The listing builds one solid part. Answer for the finished solid, in the listing's coordinates (mm). A direction names the side the tool comes from. Give positions to 0.01 mm unless a question says otherwise; leave off trailing zeros. Write each loop counter-clockwise with the first axis right and the second up, starting at its lowest first coordinate (ties: lowest second). Pieces come first, ordered by that corner, then holes. Notation, with made-up numbers: (4.5, 61.25) - (42.5, 61.25) arc R7 ccw to (42.5, 74.25) - close; hole circle Ø5 at (56, -21). An arc over 180 degrees is marked (long way). Answer in a Markdown table with one row per item. Add a question column.
from build123d import *

# Parameters (mm, degrees)
F1_DEPTH = 5
F3_DEPTH = 335
F4_W     = 5
F4_H     = 335
F5_DEPTH = 319
F7_DEPTH = 335


with BuildPart() as f1:
    # F0 (on Top) → F1 (new body)
    with BuildSketch(Plane.XY):
        Polygon((-324, 0), (0, 0), (0, 195), (-199, 195), (-199, 5), (-299, 5), (-319, 25), (-319, 195), (-324, 195), align=None)
    extrude(amount=F1_DEPTH)

    # F2 (on face) → F3 (join)
    with BuildSketch(Plane(origin=(0, 0, 0), x_dir=(1, 0, 0), z_dir=(0, 0, -1))):
        Polygon((-319, 0), (-324, 0), (-324, -195), (-319, -195), (-319, -25), align=None)
    extrude(amount=F3_DEPTH)

    # F4 (on face) → F5 (join, through all)
    with BuildSketch(Plane.YZ.offset(-319)):
        with Locations((2.5, -167.5)):
            Rectangle(F4_W, F4_H)
    extrude(amount=F5_DEPTH)

    # F6 (on face) → F7 (join, through all)
    with BuildSketch(Plane(origin=(0, 0, 0), x_dir=(1, 0, 0), z_dir=(0, 0, -1))):
        Polygon((0, -195), (0, -5), (-5, -5), (-5, -190), (-199, -190), (-199, -195), align=None)
    extrude(amount=F7_DEPTH)


solid = f1.part
1. Straight lines are drawn through the part: L1, parallel to X at y = 41.5, z = -220; L2, parallel to Y at x = -24, z = -287.5; L3, parallel to Z at x = -29, y = 83.5. For each, find the intervals that lie inside material, in ascending order. Write a range as [from, to].
2. Section A-A (y = 40) is taken. Give the vertices of the cut face in (x, z), and give its area (3 significant figures).
3. Section B-B (x = -63.5) is taken. Give the vertices of the cut face in (y, z), and give its area (4 significant figures).
4. Section D-D (x = -303.5) is taken. Give the vertices of the cut face in (y, z).
5. A tool of negligible diameter and unlimited length cuts with its end or side. For faces 1 (the face through (-309, 15, 2)), 2 (the face through (-103, 99, 0)), 3 (the face through (-139, 3, -335)), from which of +Z, -Z, +X, -X, +Y, -Y can it reach the whole face along a straight path? Write none if from no direction.
6. The mould has two halves that part along X. Classify faces 4 (the face through (-314, 11, 0)), 5 (the face through (0, 99, -163)), 6 (the face through (-164, 0, -167)): +X half, -X half, draft (parallel to the pull), parting line (faces both ways), or undercut.
7. Section C-C (z = -224.5) is taken. Give the vertices of the cut face in (x, y), and give its area (3 significant figures).
8. Given pin 1 Ø12 at (x, y) = (-123, 77.5) entering from -Z, flat-ended and moving along its own axis, determine where the tip first touches the part or whether it passes through.
Geometry check:
| question | item | result |
|---|---|---|
| 1 | L1 | [-324, -319], [-5, 0] |
| 1 | L2 | [0, 5], [190, 195] |
| 1 | L3 | [0, 5] |
| 2 | outline | (-324, -335) - (-319, -335) - (-319, 5) - (-324, 5) - close; (-199, 0) - (-5, 0) - (-5, -335) - (0, -335) - (0, 5) - (-199, 5) - close |
| 2 | area | 4,370 mm² |
| 3 | outline | (0, -335) - (5, -335) - (5, 0) - (190, 0) - (190, -335) - (195, -335) - (195, 5) - (0, 5) - close |
| 3 | area | 4,325 mm² |
| 4 | outline | (0, -335) - (5, -335) - (5, 0) - (9.5, 0) - (9.5, 5) - (0, 5) - close |
| 5 | face 1 | +Z, -Z, +Y |
| 5 | face 2 | -Z |
| 5 | face 3 | -Z, +X, -X, +Y, -Y |
| 6 | face 4 | undercut |
| 6 | face 5 | +X half |
| 6 | face 6 | draft |
| 7 | outline | (-324, 0) - (0, 0) - (0, 195) - (-199, 195) - (-199, 190) - (-5, 190) - (-5, 5) - (-319, 5) - (-319, 195) - (-324, 195) - close |
| 7 | area | 4,490 mm² |
| 8 | pin 1 | z = 0 |
